Here's how the part is built. I have some questions about the finished solid (model axes, mm). Face numbers are marked on the shaded views. Coordinates: 2 decimals unless noted, no trailing zeros. Loops run counter-clockwise (first coordinate to the right, second up) from the corner with the lowest first, then second, coordinate; pieces in that order, holes last. Notation, with made-up numbers: (-33, 81.25) -> (-7, 81.25) arc R23 cw to (-7, 89.25) -> close; hole circle Ø3 at (-25, 37.5). An arc over 180 degrees is marked (long way). Answer as a JSON object with one key per item and string values. Group by question number.
1) I'm going to push a flat-ended pin straight in: pin 1 (2 mm diameter, centred on x = 8.5, y = -7.5, fed in from -Z). Where does the tip first touch, or does it pass through?
2) I want a section at B-B (x = 6). Write out the boundary of the cut face in (y, z).
3) I need wall thicknesses on probe 1 along Y at (x, z) = (2.5, 0); probe 2 along Z at (x, y) = (2.75, 2.25); probe 3 along Z at (x, y) = (8, 3.75). Which ranges of each line are inside material? Lowest first, please. Write a range as [from, to].
4) I want a section at C-C (y = -3.5). Write out the boundary of the cut face in (x, z).
5) I want a section at D-D (z = -9). Write out the boundary of the cut face in (x, y), then the cut area to 3 significant figures.
6) I want a section at A-A (z = 0). Write out the boundary of the cut face in (x, y).
7) If we mould it in two halves opening along Z, with no side actions, what happens to the marked faces 1, 2, 3 and 4? For each: +Z half, -Z half, draft (parallel to the pull), parting line (faces both ways), or undercut.
```python
from build123d import *

# Parameters (mm, degrees)
SKETCH_1_R         = 5.1
F_01_HEX_M12_DEPTH = 10


with BuildPart() as part:
    # 草图1 → 01_HEX_M12 (new body)
    with BuildSketch(Plane(origin=(0, 0, 0), x_dir=(0, 0, -1), z_dir=(1, 0, 0))):
        Polygon((11.547005384, 0), (5.773502692, 10), (-5.773502692, 10), (-11.547005384, 0), (-5.773502692, -10), (5.773502692, -10), align=None)
        Circle(SKETCH_1_R, mode=Mode.SUBTRACT)
    extrude(amount=F_01_HEX_M12_DEPTH)


solid = part.part
```
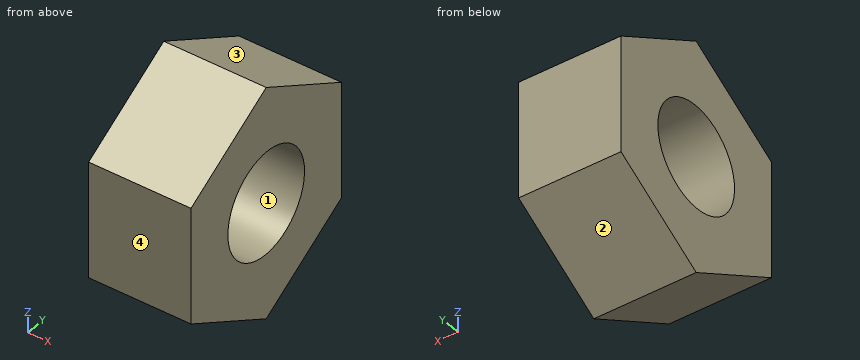
Determined:
{
 "1": {"pin 1": "z = -7.79"},
 "2": {"outline": "(-10, -5.77) -> (0, -11.55) -> (10, -5.77) -> (10, 5.77) -> (0, 11.55) -> (-10, 5.77) -> close; hole circle Ø10.2 at (0, 0)"},
 "3": {"probe 1": "[-10, -5.1], [5.1, 10]", "probe 2": "[-10.25, -4.58], [4.58, 10.25]", "probe 3": "[-9.38, -3.46], [3.46, 9.38]"},
 "4": {"outline": "(0, -9.53) -> (10, -9.53) -> (10, -3.71) -> (0, -3.71) -> close; (0, 3.71) -> (10, 3.71) -> (10, 9.53) -> (0, 9.53) -> close"},
 "5": {"outline": "(0, -4.41) -> (10, -4.41) -> (10, 4.41) -> (0, 4.41) -> close", "area": "88.2 mm^2"},
 "6": {"outline": "(0, -10) -> (10, -10) -> (10, -5.1) -> (0, -5.1) -> close; (0, 5.1) -> (10, 5.1) -> (10, 10) -> (0, 10) -> close"},
 "7": {"face 1": "undercut", "face 2": "-Z half", "face 3": "+Z half", "face 4": "draft"}
}
